Autodesk Inventor part; units mm, degrees
ref_plane "YZ Plane" through (0, 0, 0) normal (1, 0, 0) x (0, 1, 0)
ref_plane "XZ Plane" through (0, 0, 0) normal (0, 1, 0) x (-1, 0, 0)
ref_plane "XY Plane" through (0, 0, 0) normal (0, 0, 1) x (1, 0, 0)
sketch "Sketch1" plane through (0, 0, 0) normal (0, 1, 0) x (-1, 0, 0)
  circle A0 centre (33.827, -45.1473) radius 1.143
  circle A1 centre (11.7661, 26.4615) radius 1.143
  line L0 (31.3076, -49.9102) -> (7.0032, 28.9809)
  line L1 (7.0032, 28.9809) -> (55.0834, 43.7932)
  line L2 (110.1987, -25.6058) -> (31.3076, -49.9102)
  line L3 (39.3181, -47.4424) -> (15.0137, 31.4487)
  line L4 (15.0137, 31.4487) -> (7.0032, 28.9809)
  line L5 (7.0032, 28.9809) -> (31.3076, -49.9102)
  point P0 (0, 0)
  point P1 (39.8036, -47.2928)
  point P2 (15.0137, 31.4487)
  dimension "d0" = 8.382
extrude "Extrusion1" add sketch "Sketch1" along normal blind 4.064
sketch "Sketch2" plane through (0, 0, 0) normal (0, -1, 0) x (1, 0, 0)
  line L0 (-13.8437, 22.9527) -> (-33.5699, -41.0776)
  line L1 (-16.4887, 27.953) -> (-13.8437, 22.9527)
  line L2 (-33.5699, -41.0776) -> (-38.5703, -43.7227)
  line L3 (-38.3328, -44.1717) -> (-33.1464, -41.4283)
  line L4 (-33.1464, -41.4283) -> (-13.2963, 23.0042)
  line L5 (-13.2963, 23.0042) -> (-16.0397, 28.1906)
  line L6 (-39.3181, -47.4424) -> (-15.0137, 31.4487)
  line L7 (-31.3076, -49.9102) -> (-39.3181, -47.4424)
  circle A0 centre (-11.7661, 26.4615) radius 1.143
  circle A1 centre (-33.827, -45.1473) radius 1.143
  line L8 (-7.0032, 28.9809) -> (-31.3076, -49.9102)
  line L9 (-15.0137, 31.4487) -> (-7.0032, 28.9809)
  point P0 (0, 0)
  point P1 (-37.7505, -43.8637)
  point P2 (-15.7317, 27.6083)
  point P3 (-16.0256, 28.164)
  point P4 (-38.3061, -44.1576)
  dimension "d3" = 0.508
extrude "Extrusion2" add sketch "Sketch2" along normal blind 3.175 contours L6 L9 L8 L7 L3 L4 L5
sketch "Sketch3" plane through (0, 4.064, 0) normal (0, 1, 0) x (1, 0, 0)
  circle A0 centre (-11.7661, -26.4615) radius 1.143
  circle A1 centre (-33.827, 45.1473) radius 1.143
  line L0 (-31.5846, 45.8381) -> (-32.1076, 43.5508)
  line L1 (-32.1076, 43.5508) -> (-34.3499, 42.86)
  line L2 (-34.3499, 42.86) -> (-36.0693, 44.4565)
  line L3 (-36.0693, 44.4565) -> (-35.5464, 46.7439)
  line L4 (-35.5464, 46.7439) -> (-33.3041, 47.4347)
  line L5 (-33.3041, 47.4347) -> (-31.5846, 45.8381)
  line L6 (-9.5237, -25.7707) -> (-10.0466, -28.058)
  line L7 (-10.0466, -28.058) -> (-12.289, -28.7488)
  line L8 (-12.289, -28.7488) -> (-14.0084, -27.1523)
  line L9 (-14.0084, -27.1523) -> (-13.4855, -24.8649)
  line L10 (-13.4855, -24.8649) -> (-11.2431, -24.1741)
  line L11 (-11.2431, -24.1741) -> (-9.5237, -25.7707)
  line L12 (-31.3076, 49.9102) -> (-39.3181, 47.4424)
  point P0 (0, 0)
  point P1 (-38.8933, 47.5732)
  dimension "d6" = 4.064
  dimension "d7" = 4.064
extrude "Extrusion3" cut sketch "Sketch3" against normal blind 1.5875 contours A0 | L0 L1 L2 L3 L4 L5 | L6 L7 L8 L9 L10 L11
properties part number "3010 MOUNT PLATE RETAINER"
For this review, take the finished solid that the model builds, in its own axes (mm). A direction names the side the tool comes from. Coordinates: 2 decimals unless noted, no trailing zeros. Loops run counter-clockwise (first coordinate to the right, second up) from the corner with the lowest first, then second, coordinate; pieces in that order, holes last.
1. Add section D-D, the plane y = -0.75. Give the boundary of the cut face in (x, z).
2. Add section A-A, the plane y = 3.25. Give the boundary of the cut face in (x, z), then the cut area to 3 significant figures.
3. Mouldability with a two-part tool opening along X and no side actions: class faces 1 (the flat face through (-35, 2.476, -46)), 2 (the flat face through (-24, 4.064, -9)), 3 (the flat face through (-35.76, -1.57, -42.81)) as +X half, -X half, draft (parallel to the pull), parting line (faces both ways), or undercut.
4. For faces 4 (the flat face through (-14.642, -1.565, 25.548)), 5 (the flat face through (-19.326, 0.394, -11.017)), 6 (the flat face through (-12.38, 3.281, 24.524)), list the 3-axis set-ups (+Z, -Z, +X, -X, +Y, -Y) from which the entire face can be reached by the end or side of a thin tool; tool diameter is ignored.
5. Add section C-C, the plane z = 15. Give the boundary of the cut face in (x, y) (3 decimals).
6. Insertion check: P1, Ø4, axis at y = 2, z = -32, coming from the +X side; P2, Ø3, axis at y = 1.5, z = -26, coming from the -X side; P3, Ø3.5, axis at x = -11.77, z = 26.46, coming from the +Y side. Each pin has a flat end and moves straight along its axis. Give the tip position at first contact, or say it passes through.
7. Add section B-B, the plane x = -26. Give the boundary of the cut face in (y, z) (3 decimals), then the cut area to 3 significant figures.
8. For line 1 (Y direction, x = -19, z = 17.5); line 2 (X direction, y = 1.25, z = -44.5); line 3 (X direction, y = 2.5, z = 7), list the stretches that pass through material, from the lowest coordinate up.
Result:
1. outline: (-39.32, -47.44) - (-31.31, -49.91) - (-7, 28.98) - (-15.01, 31.45) - (-16.03, 28.16) - (-13.3, 23) - (-33.15, -41.43) - (-38.31, -44.16) - close; hole circle Ø2.29 at (-33.83, -45.15); hole circle Ø2.29 at (-11.77, 26.46)
2. outline: (-39.32, -47.44) - (-31.31, -49.91) - (-7, 28.98) - (-15.01, 31.45) - close; hole (-36.07, -44.46) - (-35.55, -46.74) - (-33.3, -47.43) - (-31.58, -45.84) - (-32.11, -43.55) - (-34.35, -42.86) - close; hole (-14.01, 27.15) - (-13.49, 24.86) - (-11.24, 24.17) - (-9.52, 25.77) - (-10.05, 28.06) - (-12.29, 28.75) - close
2. area: 663 mm2
3. face 1: undercut
3. face 2: draft
3. face 3: -X half
4. face 4: -X, -Y
4. face 5: -Z, +X, +Y, -Y
4. face 6: +Y
5. outline: (-20.081, 0) - (-15.762, 0) - (-15.762, -3.175) - (-11.31, -3.175) - (-11.31, 4.064) - (-20.081, 4.064) - close
6. P1: stops at x = -25.17
6. P2: stops at x = -33.17
6. P3: stops at y = 2.48
7. outline: (-3.175, -32.682) - (4.064, -32.682) - (4.064, -4.212) - (0, -4.212) - (0, -18.231) - (-3.175, -18.231) - close
7. area: 162 mm2
8. line 1: y = 0 to 4.06
8. line 2: x = -38.41 to -34.77, -32.88 to -29.64
8. line 3: x = -22.55 to -13.77
